Part model, mm, in its own coordinate system. Give positions to 0.01 mm unless a question says otherwise; leave off trailing zeros. Write each loop counter-clockwise with the first axis right and the second up, starting at its lowest first coordinate (ties: lowest second). Pieces come first, ordered by that corner, then holes. Notation, with made-up numbers: M 8,38.5 L 67,38.5 A35 ccw 67,73.5 Z; hole C 41.25,80.5 d2. An arc over 180 degrees is marked long. Answer as CSV lines item,"result". Start each with the question number.
Item 1: Pin check, flat tips, straight feed: pin 1 (5.5 mm diameter, centred on x = 5.5, y = 4, fed in from +Z); pin 2 (3.5 mm diameter, centred on y = 8.5, z = 14.5, fed in from -X); pin 3 (3.5 mm diameter, centred on x = 10.5, y = 7.5, fed in from -Z); pin 4 (0.8 mm diameter, centred on y = 0.5, z = 17.5, fed in from -X). Stop position of each tip, or through.
Item 2: Wall check: L1, parallel to Z at x = 8, y = 3.75; L2, parallel to Y at x = 0.5, z = 23.5; L3, parallel to Z at x = 6.5, y = 10.75. Give the ranges that are in metal, low to high. Write a range as from..to.
Item 3: Band-saw the part on B-B, the plane y = 2. List the corners of the cut face in (x, z), then the cut area to 3 significant figures.
Item 4: Band-saw the part on D-D, the plane z = 5.5. List the corners of the cut face in (x, y), then the cut area to 3 significant figures.
Item 5: Band-saw the part on A-A, the plane x = 10.5. List the corners of the cut face in (y, z), then the cut area to 3 significant figures.
Item 6: Band-saw the part on C-C, the plane z = -7.5. List the corners of the cut face in (x, y), then the cut area to 3 significant figures.
from build123d import *

# Parameters (mm, degrees)
F0_W      = 19.812
F0_H      = 11.43
F1_DEPTH  = 1.27
F2_T      = -0.254
F3_W      = 0.762
F3_H      = 0.762
F4_DEPTH  = 25.4
F5_W      = 0.762
F5_H      = 1.27
F6_DEPTH  = 0.762
F7_W      = 0.762
F7_H      = 0.762
F8_DEPTH  = 19.05
F9_W      = 0.762
F9_H      = 0.762
F10_DEPTH = 20.574
F11_W     = 0.762
F11_H     = 0.762
F12_DEPTH = 19.558
F14_D     = 0.127


with BuildPart() as f1:
    # F0 (on Top) → F1 (new body)
    with BuildSketch(Plane.XY):
        with Locations((9.906, 5.715)):
            Rectangle(F0_W, F0_H)
    extrude(amount=F1_DEPTH)

    # F2
    f2_openings = [f1.faces().sort_by_distance(p)[0] for p in [
        (9.906, 5.715, 0),
    ]]
    offset(amount=F2_T, openings=f2_openings)

    # F3 (on face) → F4 (join)
    with BuildSketch(Plane.XY.offset(1.27)):
        with Locations((19.431, 0.381)):
            Rectangle(F3_W, F3_H)
        with Locations((19.431, 11.049)):
            Rectangle(F3_W, F3_H)
        with Locations((0.381, 11.049)):
            Rectangle(F3_W, F3_H)
        with Locations((0.381, 0.381)):
            Rectangle(F3_W, F3_H)
    extrude(amount=F4_DEPTH)

    # F5 (on face) → F6 (join)
    with BuildSketch(Plane.YZ.offset(19.812)):
        with Locations((3.614489, 0.635)):
            Rectangle(F5_W, F5_H)
    extrude(amount=F6_DEPTH)

    # F7 (on face) → F8 (join)
    with BuildSketch(Plane(origin=(0, 0, 0), x_dir=(1, 0, 0), z_dir=(0, 0, -1))):
        with Locations((20.193, -3.614489)):
            Rectangle(F7_W, F7_H)
    extrude(amount=F8_DEPTH)

    # F9 (on face) → F10 (join)
    with BuildSketch(Plane(origin=(19.812, 0, 0), x_dir=(0, -1, 0), z_dir=(-1, 0, 0))):
        with Locations((-3.614489, -18.669)):
            Rectangle(F9_W, F9_H)
    extrude(amount=F10_DEPTH)

    # F11 (on face) → F12 (join)
    with BuildSketch(Plane.XY.offset(-18.288)):
        with Locations((-0.381, 3.614489)):
            Rectangle(F11_W, F11_H)
    extrude(amount=F12_DEPTH)

    # F14 (through all)
    with Locations(Plane.XZ.offset(-3.233489)):
        with Locations((9.906, -18.653618)):
            Hole(F14_D / 2)


solid = f1.part
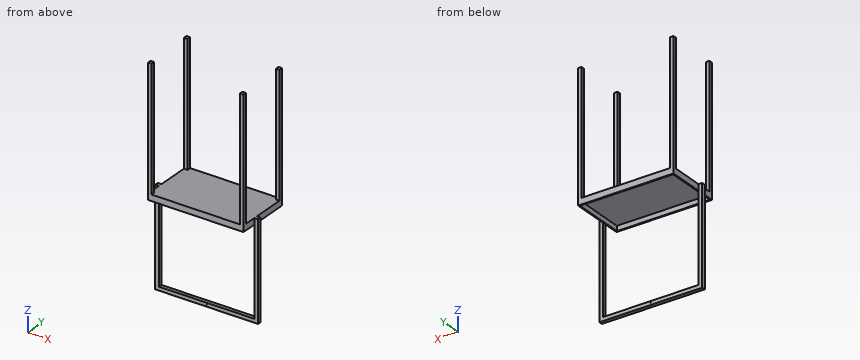
Output:
1,pin 1,"z = 1.27"
1,pin 2,"through"
1,pin 3,"z = 1.02"
1,pin 4,"x = 0"
2,L1,"-19.05..-18.29, 1.02..1.27"
2,L2,"0..0.76, 10.67..11.43"
2,L3,"1.02..1.27"
3,outline,"M 0,0 L 0.25,0 L 0.25,1.02 L 19.56,1.02 L 19.56,0 L 19.81,0 L 19.81,1.27 L 0,1.27 Z"
3,area,"5.55 mm²"
4,outline,"M 0,0 L 0.76,0 L 0.76,0.76 L 0,0.76 Z; M 0,10.67 L 0.76,10.67 L 0.76,11.43 L 0,11.43 Z; M 19.05,0 L 19.81,0 L 19.81,0.76 L 19.05,0.76 Z; M 19.05,10.67 L 19.81,10.67 L 19.81,11.43 L 19.05,11.43 Z"
4,area,"2.32 mm²"
5,outline,"M 0,0 L 0.25,0 L 0.25,1.02 L 11.18,1.02 L 11.18,0 L 11.43,0 L 11.43,1.27 L 0,1.27 Z; M 3.23,-19.05 L 4,-19.05 L 4,-18.29 L 3.23,-18.29 Z"
5,area,"4.00 mm²"
6,outline,"M -0.76,3.23 L 0,3.23 L 0,4 L -0.76,4 Z; M 19.81,3.23 L 20.57,3.23 L 20.57,4 L 19.81,4 Z"
6,area,"1.16 mm²"
